from build123d import *

# Parameters (mm, degrees)
BOSS_EXTRUDE1_DEPTH = 1.27
FILLET1_START       = -1
FILLET1_DEPTH       = 3
FILLET2_START       = -1
FILLET2_DEPTH       = 3
FILLET3_R           = 5.08
FILLET4_R           = 5.08
SKETCH3_R           = 1.5875
CUT_EXTRUDE1_DEPTH  = 39.269062151


with BuildPart() as part:
    # Sketch1 → Boss-Extrude1 (new body)
    with BuildSketch(Plane.XY):
        with BuildLine():
            add(Edge.make_bspline(
                [(-26.078451224, -26.078451224), (-25.595030672, -26.46689269), (-16.201372292, -29.50543677), (0, -7.636650328), (16.201372291, -29.50543677), (25.595030672, -26.46689269), (26.078451224, -26.078451224)],
                knots=[0.032766754, 0.032766754, 0.032766754, 0.032766754, 0.065533508, 0.5, 0.934466492, 0.967233246, 0.967233246, 0.967233246, 0.967233246], degree=3))
            add(Edge.make_bspline(
                [(26.078451224, -26.078451224), (26.46689269, -25.595030672), (29.505436772, -16.201372289), (7.636650328, -2e-09), (29.505436768, 16.201372294), (26.46689269, 25.595030672), (26.078451224, 26.078451224)],
                knots=[0.032766754, 0.032766754, 0.032766754, 0.032766754, 0.065533508, 0.5, 0.934466492, 0.967233246, 0.967233246, 0.967233246, 0.967233246], degree=3))
            add(Edge.make_bspline(
                [(-26.078451224, 26.078451224), (-25.595030672, 26.46689269), (-16.201372292, 29.50543677), (0, 7.636650328), (16.201372291, 29.50543677), (25.595030672, 26.46689269), (26.078451224, 26.078451224)],
                knots=[0.032766754, 0.032766754, 0.032766754, 0.032766754, 0.065533508, 0.5, 0.934466492, 0.967233246, 0.967233246, 0.967233246, 0.967233246], degree=3))
            add(Edge.make_bspline(
                [(-26.078451224, -26.078451224), (-26.46689269, -25.595030672), (-29.50543677, -16.201372292), (-7.636650328, 0), (-29.50543677, 16.201372291), (-26.46689269, 25.595030672), (-26.078451224, 26.078451224)],
                knots=[0.032766754, 0.032766754, 0.032766754, 0.032766754, 0.065533508, 0.5, 0.934466492, 0.967233246, 0.967233246, 0.967233246, 0.967233246], degree=3))
        make_face()
    extrude(amount=BOSS_EXTRUDE1_DEPTH)

    # Fillet1: read off the stored shape, not the designer's step
    # Fillet1 outline → Fillet1 (cut)
    with BuildSketch(Plane.XY.offset(FILLET1_START)):
        with BuildLine():
            add(Edge.make_bspline(
                [(26.078451224, 26.078451224), (25.595030672, 26.46689269), (24.088787806, 26.954113447), (22.608220096, 27.071858625), (21.782533291, 27.042115453)],
                knots=[0.032766754, 0.032766754, 0.032766754, 0.032766754, 0.065533508, 0.1076861, 0.1076861, 0.1076861, 0.1076861], degree=3))
            ThreePointArc((21.782533291, 27.042115453), (25.557510624, 25.557510623), (27.042115452, 21.78253329))
            add(Edge.make_bspline(
                [(27.042115452, 21.78253329), (27.071858625, 22.608220095), (26.954113447, 24.088787806), (26.46689269, 25.595030672), (26.078451224, 26.078451224)],
                knots=[0.8923139, 0.8923139, 0.8923139, 0.8923139, 0.934466492, 0.967233246, 0.967233246, 0.967233246, 0.967233246], degree=3))
        make_face()
    extrude(amount=FILLET1_DEPTH, mode=Mode.SUBTRACT)

    # Fillet2: read off the stored shape, not the designer's step
    # Fillet2 outline → Fillet2 (cut)
    with BuildSketch(Plane.XY.offset(FILLET2_START)):
        with BuildLine():
            add(Edge.make_bspline(
                [(-26.078451224, -26.078451224), (-25.595030672, -26.46689269), (-24.088787806, -26.954113447), (-22.608220096, -27.071858625), (-21.782533291, -27.042115453)],
                knots=[0.032766754, 0.032766754, 0.032766754, 0.032766754, 0.065533508, 0.1076861, 0.1076861, 0.1076861, 0.1076861], degree=3))
            ThreePointArc((-21.782533291, -27.042115453), (-25.557510624, -25.557510624), (-27.042115453, -21.782533291))
            add(Edge.make_bspline(
                [(-27.042115453, -21.782533291), (-27.071858625, -22.608220096), (-26.954113447, -24.088787806), (-26.46689269, -25.595030672), (-26.078451224, -26.078451224)],
                knots=[0.8923139, 0.8923139, 0.8923139, 0.8923139, 0.934466492, 0.967233246, 0.967233246, 0.967233246, 0.967233246], degree=3))
        make_face()
    extrude(amount=FILLET2_DEPTH, mode=Mode.SUBTRACT)

    # Fillet3
    fillet3_edges = [part.edges().sort_by_distance(p)[0] for p in [
        (-26.078451224, 26.078451224, 0.635),
    ]]
    fillet(fillet3_edges, radius=FILLET3_R)

    # Fillet4
    fillet4_edges = [part.edges().sort_by_distance(p)[0] for p in [
        (26.078451224, -26.078451224, 0.635),
    ]]
    fillet(fillet4_edges, radius=FILLET4_R)

    # Sketch3 → Cut-Extrude1 (cut, through all)
    with BuildSketch(Plane.XY.offset(1.27)):
        with Locations((-21.911824935, 21.911824935)):
            Circle(SKETCH3_R)
        with Locations((21.911824935, 21.911824935)):
            Circle(SKETCH3_R)
        with Locations((21.911824935, -21.911824935)):
            Circle(SKETCH3_R)
        with Locations((-21.911824935, -21.911824935)):
            Circle(SKETCH3_R)
        with BuildLine():
            add(Edge.make_bspline(
                [(-7.336925612, -7.336925612), (-7.094564954, -7.539990493), (-4.441685448, -8.467510629), (0, -2.70941912), (4.441685448, -8.467510629), (7.094564954, -7.539990493), (7.336925612, -7.336925612)],
                knots=[0.055321023, 0.055321023, 0.055321023, 0.055321023, 0.110642047, 0.5, 0.889357953, 0.944678976, 0.944678976, 0.944678976, 0.944678976], degree=3))
            add(Edge.make_bspline(
                [(7.336925612, 7.336925612), (7.539990493, 7.094564954), (8.467510629, 4.441685448), (2.70941912, 0), (8.467510629, -4.441685448), (7.539990493, -7.094564954), (7.336925612, -7.336925612)],
                knots=[0.055321023, 0.055321023, 0.055321023, 0.055321023, 0.110642047, 0.5, 0.889357953, 0.944678977, 0.944678977, 0.944678977, 0.944678977], degree=3))
            add(Edge.make_bspline(
                [(-7.336925612, 7.336925612), (-7.094564954, 7.539990493), (-4.441685448, 8.467510629), (0, 2.70941912), (4.441685448, 8.467510629), (7.094564954, 7.539990493), (7.336925612, 7.336925612)],
                knots=[0.055321023, 0.055321023, 0.055321023, 0.055321023, 0.110642047, 0.5, 0.889357953, 0.944678977, 0.944678977, 0.944678977, 0.944678977], degree=3))
            add(Edge.make_bspline(
                [(-7.336925612, 7.336925612), (-7.539990493, 7.094564954), (-8.467510629, 4.441685448), (-2.70941912, 0), (-8.467510629, -4.441685448), (-7.539990493, -7.094564954), (-7.336925612, -7.336925612)],
                knots=[0.055321023, 0.055321023, 0.055321023, 0.055321023, 0.110642047, 0.5, 0.889357953, 0.944678977, 0.944678977, 0.944678977, 0.944678977], degree=3))
        make_face()
    extrude(amount=-CUT_EXTRUDE1_DEPTH, mode=Mode.SUBTRACT)


solid = part.part
The listing builds one solid part. Answer for the finished solid, in the listing's coordinates (mm). Coordinates: 2 decimals unless noted, no trailing zeros. Answer in a Markdown table with one row per item. Add a question column.
Item 1: Find the intervals of material crossed by L1, parallel to Y at x = 23, z = 0.4; L2, parallel to Y at x = -6, z = 0.5; L3, parallel to Y at x = -22, z = 0.3, in increasing order. Write a range as from..to.
Item 2: Find section A-A (z = 0.8). State how many separate pieces and enclosed holes the cut face has, then the cut area to 3 significant figures.
Item 3: Determine the mould class of faces 1 (the face through (-21.06, -20.57, 0.64)), 2 (the face through (0, -6, 0)), 3 (the face through (20.74, 22.98, 0.64)) for opening direction X: +X half, -X half, draft (parallel to the pull), parting line (faces both ways), or undercut.
Result set:
| question | item | result |
|---|---|---|
| 1 | L1 | y = -26.94..-23.07, -20.76..-11.47, 11.47..20.76, 23.07..26.94 |
| 1 | L2 | y = -19.86..-7.75, -1.93..1.93, 7.75..19.86 |
| 1 | L3 | y = -27.05..-23.5, -20.33..-9.82, 9.82..20.33, 23.5..27.05 |
| 2 | separate pieces | 1 |
| 2 | enclosed holes | 5 |
| 2 | area | 1,920 mm² |
| 3 | face 1 | undercut |
| 3 | face 2 | draft |
| 3 | face 3 | undercut |
